Geometry check sheet. Reference: the model listing, model coordinates, mm. A direction names the side the tool comes from. Round coordinates to 2 decimals unless told otherwise and drop trailing zeros. Order: outer loops, then holes, each group sorted by start corner. A loop starts at its lowest first (then second) coordinate and runs counter-clockwise, first axis right, second up. Notation, with made-up numbers: (34.25, 78) -> (59.25, 78) arc R18 ccw to (59.25, 91) -> close; hole circle Ø11 at (41, 85.25). An arc over 180 degrees is marked (long way). Use a Markdown table: item, result. Add a question column.
Item 1: Mould release check, pull along X, two halves, no side actions. Record for faces 1 (the flat face through (66.84, -12.52, 5.01)), 2 (the flat face through (-7.464, -12.522, 4.876)), 3 (the flat face through (-61.934, -12.522, 5.015)), 4 (the flat face through (81.69, -12.52, 4.88)): pulls with the +X half, pulls with the -X half, needs draft (parallel to the pull), parting line crosses it, or undercut.
Item 2: Gauge pin test, flat ends, axial feed: pin 1 Ø3 at (x, y) = (-9.5, -16.5) entering from +Z; pin 2 Ø8 at (x, y) = (4.5, -5.5) entering from +Z. Record the tip position at first contact, or that the pin passes through.
Item 3: Set-up check for faces 5 (the flat face through (84.221, -13, -8)), 6 (the flat face through (-2.5, -12.52, 5.01)): record each of +Z, -Z, +X, -X, +Y, -Y from which the full face is reachable in a straight line by a thin tool's end or side.
Item 4: Sectioned sample at B-B, the plane x = 62.5. Record the cut outline in (y, z), and give its area (3 significant figures).
Item 5: Material ranges on probe 1 along Z at (x, y) = (-9, -6.75); probe 2 along Z at (x, y) = (55.5, -18.25), recorded low to high. Write a range as [from, to].
Item 6: Sectioned sample at A-A, the plane z = 1.5. State how many separate pieces and enclosed holes the cut face has, and give its area (3 significant figures).
Item 7: Sectioned sample at D-D, the plane x = 7. Record the cut outline in (y, z).
from build123d import *

# Parameters (mm, degrees)
F1_DEPTH = 25.4


with BuildPart() as f1:
    # F0 (on Front) → F1 (new body)
    with BuildSketch(Plane.XZ):
        Polygon((54.433102, 0), (64.313702, 0), (59.373402, 9.891078), align=None)
        Polygon((44.527102, 0), (54.407702, 0), (49.467402, 9.891078), align=None)
        Polygon((34.621102, 0), (44.501702, 0), (39.561402, 9.891078), align=None)
        Polygon((24.715102, 0), (34.595702, 0), (29.655402, 9.891078), align=None)
        Polygon((19.749402, 9.891078), (14.809102, 0), (24.689702, 0), align=None)
        Polygon((9.843402, 9.891078), (4.903102, 0), (14.783702, 0), align=None)
        Polygon((-0.062598, 9.891078), (-5.002898, 0), (4.877702, 0), align=None)
        Polygon((-9.968598, 9.891078), (-14.908898, 0), (-5.028298, 0), align=None)
        Polygon((-19.874598, 9.891078), (-24.814898, 0), (-14.934298, 0), align=None)
        Polygon((-29.780598, 9.891078), (-34.720898, 0), (-24.840298, 0), align=None)
        Polygon((-39.686598, 9.891078), (-44.626898, 0), (-34.746298, 0), align=None)
        Polygon((-49.592598, 9.891078), (-54.532898, 0), (-44.652298, 0), align=None)
        Polygon((-59.498598, 9.891078), (-64.438898, 0), (-54.558298, 0), align=None)
        Polygon((74.245102, 0), (84.125702, 0), (79.185402, 9.891078), align=None)
        Polygon((64.339102, 0), (74.219702, 0), (69.279402, 9.891078), align=None)
        Polygon((-54.558298, 0), (-64.438898, 0), (-64.438898, -16.354553), (84.22105, -16.354553), (84.22105, 0), (84.125702, 0), (74.245102, 0), (74.219702, 0), (64.339102, 0), (64.313702, 0), (54.433102, 0), (54.407702, 0), (44.527102, 0), (44.501702, 0), (34.621102, 0), (34.595702, 0), (24.715102, 0), (24.689702, 0), (14.809102, 0), (14.783702, 0), (4.903102, 0), (4.877702, 0), (-5.002898, 0), (-5.028298, 0), (-14.908898, 0), (-14.934298, 0), (-24.814898, 0), (-24.840298, 0), (-34.720898, 0), (-34.746298, 0), (-44.626898, 0), (-44.652298, 0), (-54.532898, 0), align=None)
    extrude(amount=F1_DEPTH)


solid = f1.part
Found:
| question | item | result |
|---|---|---|
| 1 | face 1 | undercut |
| 1 | face 2 | undercut |
| 1 | face 3 | pulls with the -X half |
| 1 | face 4 | pulls with the +X half |
| 2 | pin 1 | stops at z = 9.89 |
| 2 | pin 2 | stops at z = 8.76 |
| 3 | face 5 | +Z, -Z, +X, +Y, -Y |
| 3 | face 6 | +Z, +Y, -Y |
| 4 | outline | (-25.4, -16.35) -> (0, -16.35) -> (0, 3.63) -> (-25.4, 3.63) -> close |
| 4 | area | 508 mm2 |
| 5 | probe 1 | z = [-16.35, 7.95] |
| 5 | probe 2 | z = [-16.35, 2.14] |
| 6 | separate pieces | 15 |
| 6 | enclosed holes | 0 |
| 6 | area | 3,190 mm2 |
| 7 | outline | (-25.4, -16.35) -> (0, -16.35) -> (0, 4.2) -> (-25.4, 4.2) -> close |
